The figure shows three views and two pictorial views of one solid part (mm, origin at its lowest corner). Answer the questions. Round coordinates to 2 decimals unless told otherwise and drop trailing zeros. Write each loop counter-clockwise with the first axis right and the second up, starting at its lowest first coordinate (ties: lowest second). Pieces come first, ordered by that corner, then holes.
Item 1: This flat-tipped pin is pushed along its axis until it touches: pin 1 (1.5 mm diameter, centred on x = 34, y = 24.5, fed in from +Z). Where does it stop, or does it pass through?
Item 2: Find the intervals of material crossed by probe 1 along Z at (x, y) = (20, 43); probe 2 along Z at (x, y) = (6, 51); probe 3 along Y at (x, z) = (9.5, 8.25), in increasing order.
Item 3: Find section A-A on z = 10. Give the vertices of the cut face in (x, y).
Item 4: Find section C-C on x = 27. Give the vertices of the cut face in (y, z).
Item 5: Find section D-D on z = 4.5. Give the vertices of the cut face in (x, y), then the cut area to 3 significant figures.
Item 6: Find section B-B on y = 26.5. Give the vertices of the cut face in (x, z), then the cut area to 3 significant figures.
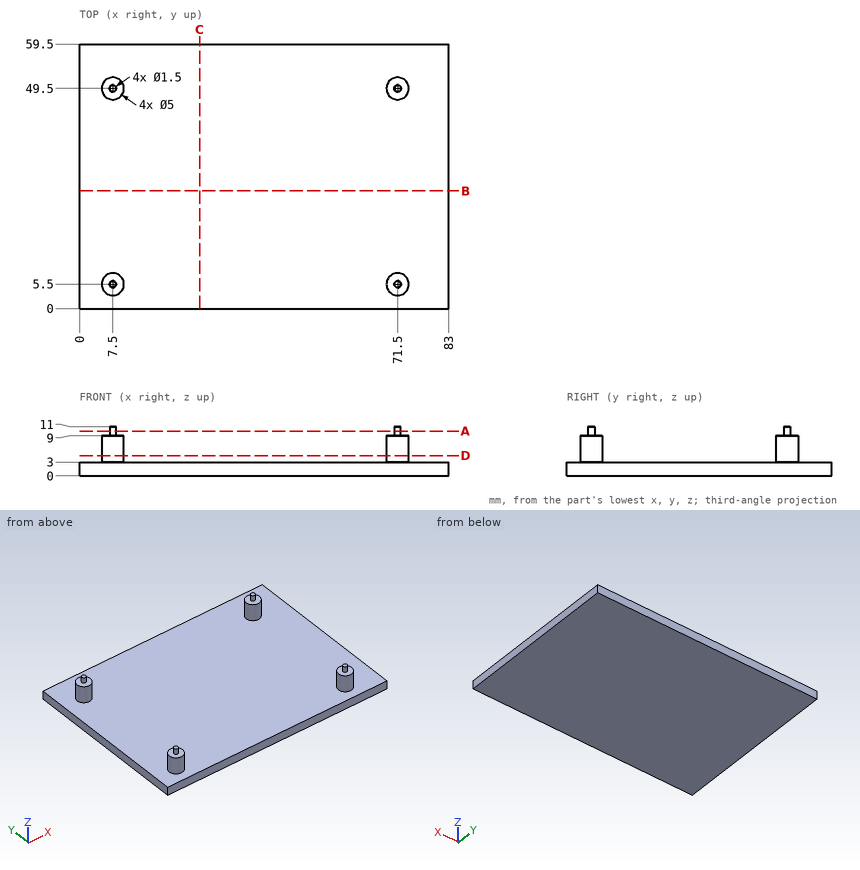
Check values:
1. pin 1: stops at z = 3
2. probe 1: z = 0 to 3
2. probe 2: z = 0 to 9
2. probe 3: y = 4 to 7, 48 to 51
3. outline: circle Ø1.5 at (7.5, 5.5); circle Ø1.5 at (7.5, 49.5); circle Ø1.5 at (71.5, 5.5); circle Ø1.5 at (71.5, 49.5)
4. outline: (0, 0) - (59.5, 0) - (59.5, 3) - (0, 3) - close
5. outline: circle Ø5 at (7.5, 5.5); circle Ø5 at (7.5, 49.5); circle Ø5 at (71.5, 5.5); circle Ø5 at (71.5, 49.5)
5. area: 78.5 mm2
6. outline: (0, 0) - (83, 0) - (83, 3) - (0, 3) - close
6. area: 249 mm2
